Input: part model. Units: mm. Frame: model coordinates. A direction names the side the tool comes from. Round coordinates to 2 decimals unless told otherwise and drop trailing zeros. Loops run counter-clockwise (first coordinate to the right, second up) from the corner with the lowest first, then second, coordinate; pieces in that order, holes last. Notation, with made-up numbers: (-38, 4) -> (-7, 4) arc R16 cw to (-7, 34) -> close; hole circle Ø7 at (-32.5, -15.5). An arc over 180 degrees is marked (long way). Answer in a Markdown table with one row per item. Add a question column.
Q1. Section D-D, the plane z = 12.7. Output: boundary loops of the cut face in (x, y).
Q2. Ray query, L1, parallel to Y at x = 25, z = 6; L2, parallel to Y at x = 24.5, z = 17; L3, parallel to X at y = 29, z = 13.25. Return the intervals inside material, ascending. Write a range as from..to.
Q3. Mould query, pull axis Z, two halves, no side actions, for faces 6 (the face through (-42.122, 3.615, 13.451)), 7 (the face through (-41, 0, 13)), 8 (the face through (19, 27, 17.4)). Classes: pulls with the +Z half, pulls with the -Z half, needs draft (parallel to the pull), parting line crosses it, or undercut.
Q4. Section B-B, the plane x = 25. Output: boundary loops of the cut face in (y, z), and give its area (3 significant figures).
Q5. Reachability of faces 1 (the face through (-46.39, 42.58, 12.52)), 2 (the face through (-1, 28, 0)), 3 (the face through (36.085, 24.404, 21.456)), 4 (the face through (35.51, 6.08, 12.52)), 5 (the face through (31.45, 18.88, 3.94)) from +Z, -Z, +X, -X, +Y, -Y: full face, straight path, thin tool, end or side. Return the list, or none.
Q6. Pin query (flat end, axial travel): pin 1 (6 mm diameter, centred on x = 23, z = 11.5, fed in from -Y); pin 2 (1.5 mm diameter, centred on x = -29, y = 15, fed in from -Z); pin 3 (19 mm diameter, centred on x = 26, y = 31, fed in from +Z); pin 4 (7 mm diameter, centred on x = 22, y = 23, fed in from -Z). Return the tip coordinate at first contact, or that it passes through.
Q7. Section C-C, the plane z = 18.75. Output: boundary loops of the cut face in (x, y), and give its area (3 significant figures).
Q8. Section A-A, the plane y = 29. Output: boundary loops of the cut face in (x, z), and give its area (3 significant figures).
```python
from build123d import *

# Parameters (mm, degrees)
SKETCH002_R     = 6
PAD_DEPTH       = 25.4
SKETCH_R        = 12
POCKET_DEPTH    = 8
SKETCH003_R     = 12
POCKET001_DEPTH = 8
SKETCH004_R     = 2.5
POCKET002_DEPTH = 16


with BuildPart() as part:
    # Sketch002 → Pad (new body)
    with BuildSketch(Plane.XY):
        with BuildLine():
            Line((-32, 0), (-38.928203, 12))
            Line((-38.928203, 12), (38.928203, 12))
            Line((38.928203, 12), (32, 0))
            Line((50, 0), (32, 0))
            Line((50, 33.999968), (50, 0))
            ThreePointArc((50, 33.999968), (46.485286, 42.485276), (37.999982, 46))
            Line((-37.999961, 45.999976), (37.999982, 46))
            ThreePointArc((-37.999961, 45.999976), (-46.485271, 42.485268), (-50, 33.999968))
            Line((-50, 0), (-50, 33.999968))
            Line((-32, 0), (-50, 0))
        make_face()
        with Locations((25, 29)):
            Circle(SKETCH002_R, mode=Mode.SUBTRACT)
    extrude(amount=PAD_DEPTH)

    # Sketch → Pocket (cut)
    with BuildSketch(Plane.XY.offset(25.4)):
        with Locations((25, 29)):
            Circle(SKETCH_R)
    extrude(amount=-POCKET_DEPTH, mode=Mode.SUBTRACT)

    # Sketch003 → Pocket001 (cut)
    with BuildSketch(Plane(origin=(0, 0, 0), x_dir=(1, 0, 0), z_dir=(0, 0, -1))):
        with Locations((25, -29)):
            Circle(SKETCH003_R)
    extrude(amount=-POCKET001_DEPTH, mode=Mode.SUBTRACT)

    # Sketch004 → Pocket002 (cut)
    with BuildSketch(Plane(origin=(-50, 0, 0), x_dir=(0, -1, 0), z_dir=(-1, 0, 0))):
        with Locations((-6, 12.7)):
            Circle(SKETCH004_R)
    extrude(amount=-POCKET002_DEPTH, mode=Mode.SUBTRACT)


solid = part.part
```
Answer block:
| question | item | result |
|---|---|---|
| 1 | outline | (-50, 0) -> (-32, 0) -> (-34.02, 3.5) -> (-50, 3.5) -> close; (-50, 8.5) -> (-36.91, 8.5) -> (-38.93, 12) -> (38.93, 12) -> (32, 0) -> (50, 0) -> (50, 34) arc R12 ccw to (38, 46) -> (-38, 46) arc R12 ccw to (-50, 34) -> close; hole circle Ø12 at (25, 29) |
| 2 | L1 | 12..17, 41..46 |
| 2 | L2 | 12..23.02, 34.98..46 |
| 2 | L3 | -50..19, 31..50 |
| 3 | face 6 | undercut |
| 3 | face 7 | needs draft |
| 3 | face 8 | pulls with the +Z half |
| 4 | outline | (12, 0) -> (17, 0) -> (17, 8) -> (23, 8) -> (23, 17.4) -> (17, 17.4) -> (17, 25.4) -> (12, 25.4) -> close; (35, 8) -> (41, 8) -> (41, 0) -> (46, 0) -> (46, 25.4) -> (41, 25.4) -> (41, 17.4) -> (35, 17.4) -> close |
| 4 | area | 367 mm^2 |
| 5 | face 1 | +Z, -Z, -X, +Y |
| 5 | face 2 | -Z, +X, -X, +Y, -Y |
| 5 | face 3 | +Z |
| 5 | face 4 | +Z, -Z |
| 5 | face 5 | -Z |
| 6 | pin 1 | y = 12 |
| 6 | pin 2 | z = 0 |
| 6 | pin 3 | z = 17.4 |
| 6 | pin 4 | z = 8 |
| 7 | outline | (-50, 0) -> (-32, 0) -> (-38.93, 12) -> (38.93, 12) -> (32, 0) -> (50, 0) -> (50, 34) arc R12 ccw to (38, 46) -> (-38, 46) arc R12 ccw to (-50, 34) -> close; hole circle Ø24 at (25, 29) |
| 7 | area | 3,230 mm^2 |
| 8 | outline | (-50, 0) -> (13, 0) -> (13, 8) -> (19, 8) -> (19, 17.4) -> (13, 17.4) -> (13, 25.4) -> (-50, 25.4) -> close; (31, 8) -> (37, 8) -> (37, 0) -> (50, 0) -> (50, 25.4) -> (37, 25.4) -> (37, 17.4) -> (31, 17.4) -> close |
| 8 | area | 2,040 mm^2 |
